Can you work these out from the model? Positions are in its coordinate system, mm. Face numbers are marked on the shaded views. Coordinates: 2 decimals unless noted, no trailing zeros. Order: outer loops, then holes, each group sorted by start corner. A loop starts at its lowest first (then second) coordinate and runs counter-clockwise, first axis right, second up. Notation, with made-up numbers: (-29.5, -29) -> (23.5, -29) arc R8 cw to (23.5, -17) -> close; hole circle Ø9 at (77, 65). An arc over 180 degrees is marked (long way). Write item = value, one per line. Start each with the question number.
from build123d import *

# Parameters (mm, degrees)
F0_W     = 139.7
F0_H     = 88.9
F1_DEPTH = 609.6
F2_SIZE  = 63.5
F3_W     = 44.45
F3_H     = 44.003254
F4_DEPTH = 50.8


with BuildPart() as f1:
    # F0 (on Front) → F1 (new body)
    with BuildSketch(Plane.XZ):
        with Locations((69.85, 44.45)):
            Rectangle(F0_W, F0_H)
    extrude(amount=F1_DEPTH)

    # F2
    f2_edges = [f1.edges().sort_by_distance(p)[0] for p in [
        (139.7, -609.6, 44.45),
    ]]
    chamfer(f2_edges, length=F2_SIZE)

    # F3 (on face) → F4 (cut)
    with BuildSketch(Plane(origin=(342.9, -342.9, 0), x_dir=(0.707107, 0.707107, 0), z_dir=(0.707107, -0.707107, 0))):
        with Locations((-332.269476, 44.45)):
            Rectangle(F3_W, F3_H)
    extrude(amount=-F4_DEPTH, mode=Mode.SUBTRACT)


solid = f1.part
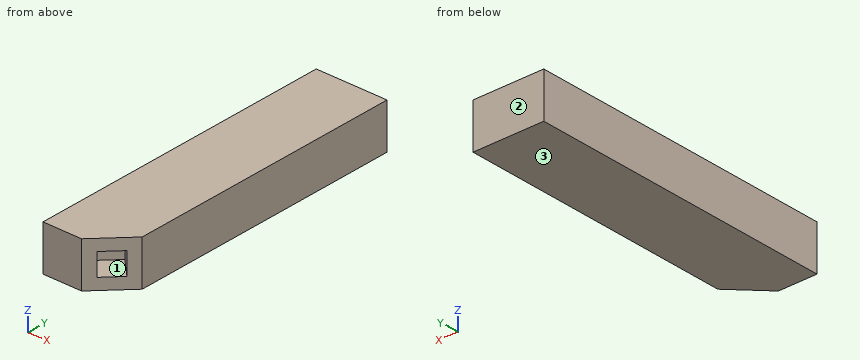
(1) If I drill on L1, parallel to Y at x = 73.5, z = 49.5; L2, parallel to Y at x = 96, z = 15.5; L3, parallel to Y at x = 100.5, z = 13, over which ranges is the centre line in solid material (lowest first)? Write a range as from..to.
(2) Imagine slicing it at A-A (z = 11). Write out the boundary of the cut face in (x, y).
(3) Imagine slicing it at C-C (y = -572.5). Write out the boundary of the cut face in (x, z), plus the area to 3 significant figures.
(4) Imagine slicing it at B-B (x = 102). Write out the boundary of the cut face in (y, z), plus the area to 3 significant figures.
(5) Thinking about a two-plate mould opening in Z: for the marked faces 1, 2 and 3, which applies, +Z half, -Z half, draft (parallel to the pull), parting line (faces both ways), or undercut?
(6) Imagine slicing it at D-D (z = 34.5). Write out the boundary of the cut face in (x, y).
Result set:
q1.L1 = -609.6..-574.83, -540.46..0
q1.L2 = -589.8..0
q1.L3 = -585.3..0
q2.outline = (0, -609.6) -> (76.2, -609.6) -> (139.7, -546.1) -> (139.7, 0) -> (0, 0) -> close
q3.outline = (0, 0) -> (113.3, 0) -> (113.3, 22.45) -> (71.17, 22.45) -> (71.17, 66.45) -> (113.3, 66.45) -> (113.3, 88.9) -> (0, 88.9) -> close
q3.area = 8,220 mm2
q4.outline = (-583.8, 0) -> (0, 0) -> (0, 88.9) -> (-583.8, 88.9) -> (-583.8, 66.45) -> (-540.47, 66.45) -> (-540.47, 22.45) -> (-583.8, 22.45) -> close
q4.area = 50,000 mm2
q5.face_1 = undercut
q5.face_2 = draft
q5.face_3 = -Z half
q6.outline = (0, -609.6) -> (76.2, -609.6) -> (92.23, -593.57) -> (56.31, -557.64) -> (87.74, -526.21) -> (123.67, -562.13) -> (139.7, -546.1) -> (139.7, 0) -> (0, 0) -> close
